```python
from build123d import *

# Parameters (mm, degrees)
F2_DEPTH = 10
F1_W     = 30
F1_H     = 130
F3_DEPTH = 5


with BuildPart() as f2:
    # F0 (on Top) → F2 (new body)
    with BuildSketch(Plane.XY):
        with BuildLine():
            Line((130, 150), (-130, 150))
            ThreePointArc((-130, 150), (-135.857864, 135.857864), (-150, 130))
            Line((-150, 130), (-150, -130))
            ThreePointArc((-150, -130), (-135.857864, -135.857864), (-130, -150))
            Line((-130, -150), (130, -150))
            ThreePointArc((130, -150), (135.857864, -135.857864), (150, -130))
            Line((150, -130), (150, 130))
            ThreePointArc((150, 130), (135.857864, 135.857864), (130, 150))
        make_face()
    extrude(amount=-F2_DEPTH)

    # F1 (on Top) → F3 (cut)
    with BuildSketch(Plane.XY):
        Polygon((-15, 20), (-20, 20), (-20, -20), (20, -20), (20, 20), (15, 20), align=None)
        with Locations((0, 85)):
            Rectangle(F1_W, F1_H)
    extrude(amount=-F3_DEPTH, mode=Mode.SUBTRACT)


solid = f2.part
```
Build history of the part. All positions in model axes, mm. Round coordinates to 2 decimals unless told otherwise and drop trailing zeros. Write each loop counter-clockwise with the first axis right and the second up, starting at its lowest first coordinate (ties: lowest second). Pieces come first, ordered by that corner, then holes. Notation, with made-up numbers: (35, -30) - (74, -30) arc R28 cw to (74, -3) - close; hole circle Ø3 at (65.25, 5.5). An arc over 180 degrees is marked (long way). Write each question's results on one line, items separated by ' | '. Start each with the question number.
Item 1: Saw through at B-B (y = 14.5). Write the cut outline in (x, z), and give its area (3 significant figures).
Item 2: Wall check: L1, parallel to X at y = 60, z = -4.25; L2, parallel to Z at x = -6.5, y = -3.5; L3, parallel to Y at x = 134, z = -9. Give the ranges that are in metal, low to high. Write a range as [from, to].
Item 3: Saw through at A-A (z = -2.5). Write the cut outline in (x, y), and give its area (3 significant figures).
Item 4: Drop flat-ended pins along their axis: P1, Ø2.5, axis at x = -10, z = -3, coming from the +Y side; P2, Ø20, axis at x = 1.5, y = 107, coming from the +Z side. Give the stop position or say it passes through.
Item 5: Saw through at C-C (y = 91.5). Write the cut outline in (x, z), and give its area (3 significant figures).
Results are:
1) outline: (-150, -10) - (150, -10) - (150, 0) - (20, 0) - (20, -5) - (-20, -5) - (-20, 0) - (-150, 0) - close | area: 2,800 mm²
2) L1: x = [-150, -15], [15, 150] | L2: z = [-10, -5] | L3: y = [-138, 138]
3) outline: (-150, -130) arc R20 cw to (-130, -150) - (130, -150) arc R20 cw to (150, -130) - (150, 130) arc R20 cw to (130, 150) - (15, 150) - (15, 20) - (20, 20) - (20, -20) - (-20, -20) - (-20, 20) - (-15, 20) - (-15, 150) - (-130, 150) arc R20 cw to (-150, 130) - close | area: 83,200 mm²
4) P1: stops at y = -20 | P2: stops at z = -5
5) outline: (-150, -10) - (150, -10) - (150, 0) - (15, 0) - (15, -5) - (-15, -5) - (-15, 0) - (-150, 0) - close | area: 2,850 mm²
